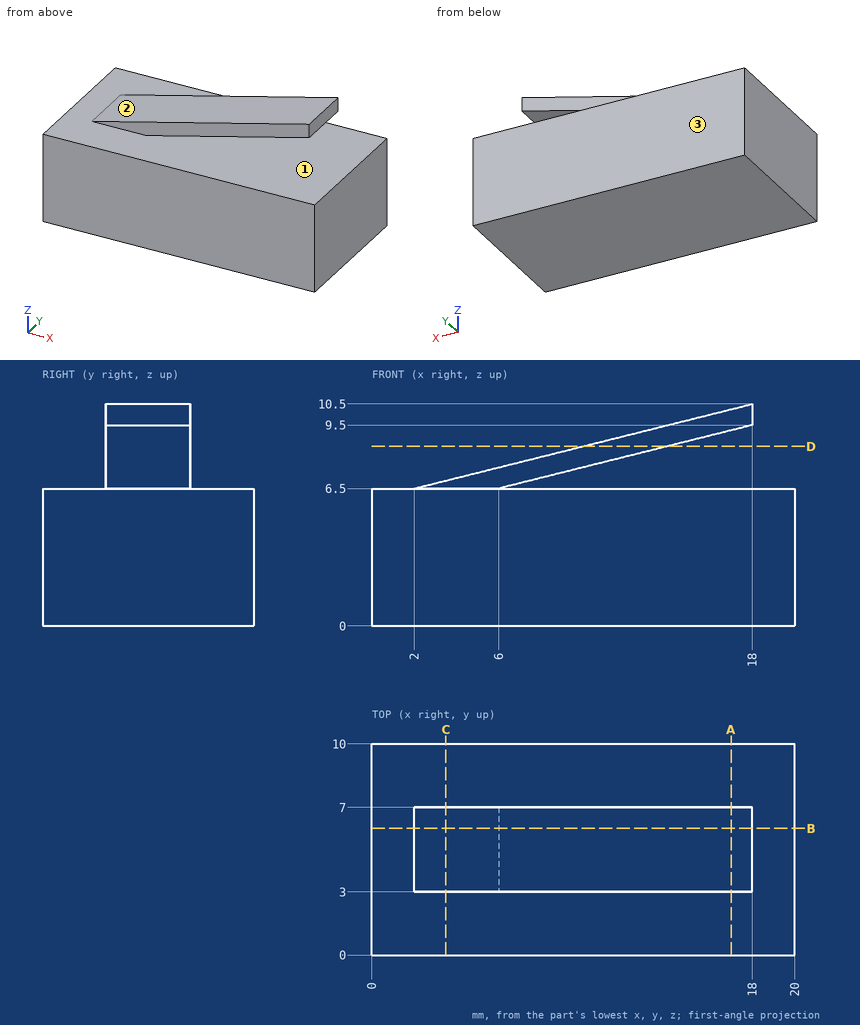
Answer from the drawing. Dimensions are ordinates in mm from the lowest x, y and z of the part. Give positions to 0.01 mm unless a question says otherwise; leave off trailing zeros. Order: outer loops, then holes, each group sorted by start corner. A loop starts at its lowest first (then second) coordinate and runs counter-clockwise, first axis right, second up.
Item 1: The part is cut by section A-A, the plane x = 17. Give the vertices of the cut face in (y, z).
From the geometry:
outline: (0, 0) - (10, 0) - (10, 6.5) - (0, 6.5) - close; (3, 9.25) - (7, 9.25) - (7, 10.25) - (3, 10.25) - close
Item 2: Find the intervals of material crossed by probe 1 along Z at (x, y) = (1.25, 1.5); probe 2 along Z at (x, y) = (17.5, 6) (3 decimals); probe 3 along Y at (x, z) = (7, 7), in increasing order.
From the geometry:
probe 1: z = 0 to 6.5
probe 2: z = 0 to 6.5, 9.375 to 10.375
probe 3: y = 3 to 7
Item 3: For a pull along Z with two mould halves and no side action, classify the marked faces 1, 2 and 3 as pulls with the +Z half, pulls with the -Z half, needs draft (parallel to the pull), parting line crosses it, or undercut.
From the geometry:
face 1: undercut
face 2: pulls with the +Z half
face 3: needs draft
Item 4: The part is cut by section B-B, the plane y = 6. Give the vertices of the cut face in (x, z).
From the geometry:
outline: (0, 0) - (20, 0) - (20, 6.5) - (6, 6.5) - (18, 9.5) - (18, 10.5) - (2, 6.5) - (0, 6.5) - close
Item 5: Given pin 1 Ø4.5 at (x, z) = (13, 9.5) entering from -Y; pin 2 Ø1.1 at (y, z) = (4.5, 10) entering from +X; pin 3 Ø2 at (x, z) = (7.5, 9) entering from +Y, each flat-ended and moving along its own axis, determine where each tip first touches the part or whether it passes through.
From the geometry:
pin 1: stops at y = 3
pin 2: stops at x = 18
pin 3: passes through
Item 6: The part is cut by section C-C, the plane x = 3.5. Give the vertices of the cut face in (y, z) (3 decimals).
From the geometry:
outline: (0, 0) - (10, 0) - (10, 6.5) - (7, 6.5) - (7, 6.875) - (3, 6.875) - (3, 6.5) - (0, 6.5) - close
Item 7: The part is cut by section D-D, the plane z = 8.5. Give the vertices of the cut face in (x, y).
From the geometry:
outline: (10, 3) - (14, 3) - (14, 7) - (10, 7) - close
